Read the model definition and answer for the solid it produces. Units are mm, in the model's axes. Coordinates: 2 decimals unless noted, no trailing zeros. Loops run counter-clockwise (first coordinate to the right, second up) from the corner with the lowest first, then second, coordinate; pieces in that order, holes last. Notation, with made-up numbers: (80, -19) - (123, -19) arc R25 cw to (123, 3) - close; hole circle Ø5 at (52, 84.25). An arc over 180 degrees is marked (long way). Use one line per item in the form item = value.
from build123d import *

# Parameters (mm, degrees)
F0_R     = 83.8
F0_R_2   = 80
F1_DEPTH = 800
F2_W     = 94.3220257759
F2_H     = 124.5050393045
F3_DEPTH = 84.8


with BuildPart() as f1:
    # F0 (on Front) → F1 (new body)
    with BuildSketch(Plane.XZ):
        Circle(F0_R)
        Circle(F0_R_2, mode=Mode.SUBTRACT)
    extrude(amount=F1_DEPTH)

    # F2 (on Top) → F3 (cut, up to face)
    with BuildSketch(Plane.XY):
        with Locations((0, -93.3787897229)):
            Rectangle(F2_W, F2_H)
    extrude(amount=-F3_DEPTH, mode=Mode.SUBTRACT)


solid = f1.part
Item 1: The part is cut by section D-D on y = -451. Give the vertices of the cut face in (x, z).
Results below:
outline = circle Ø167.6 at (0, 0); hole circle Ø160 at (0, 0)
Item 2: For a pull along Y with two mould halves and no side action, classify faces 1 (the flat face through (0, -31.126, -81)), 2 (the flat face through (31, 0, -74)), 3 (the flat face through (0, -155.631, -81)), 4 (the flat face through (31, -800, -74)) as +Y half, -Y half, draft (parallel to the pull), parting line (faces both ways), or undercut.
Results below:
face_1 = undercut
face_2 = +Y half
face_3 = undercut
face_4 = -Y half
Item 3: The part is cut by section C-C on x = 65. Give the vertices of the cut face in (y, z), plus the area to 3 significant figures.
Results below:
outline = (-800, -52.89) - (0, -52.89) - (0, -46.64) - (-800, -46.64) - close; (-800, 46.64) - (0, 46.64) - (0, 52.89) - (-800, 52.89) - close
area = 10,000 mm²
Item 4: The part is cut by section B-B on z = 0. Give the vertices of the cut face in (x, y), plus the area to 3 significant figures.
Results below:
outline = (-83.8, -800) - (-80, -800) - (-80, 0) - (-83.8, 0) - close; (80, -800) - (83.8, -800) - (83.8, 0) - (80, 0) - close
area = 6,080 mm²
Item 5: Find the intervals of material crossed by L1, parallel to Z at x = 0, y = -384; L2, parallel to X at y = -158, z = 3; L3, parallel to Y at x = -39, z = -73, in increasing order.
Results below:
L1 = -83.8 to -80, 80 to 83.8
L2 = -83.75 to -79.94, 79.94 to 83.75
L3 = -800 to -155.63, -31.13 to 0
Item 6: Each of these flat-tipped pins is pushed along its axis until it touches: P1, Ø8, axis at y = -543, z = -39, coming from the +X side; P2, Ø8, axis at y = -105, z = 54, coming from the +X side; P3, Ø4, axis at y = -576.5, z = -66, coming from the -X side. Where does it stop, or does it pass through?
Results below:
P1 = 76.14
P2 = 67.25
P3 = -54.1
Item 7: The part is cut by section A-A on x = 0. Give the vertices of the cut face in (y, z), plus the area to 3 significant figures.
Results below:
outline = (-800, -83.8) - (-155.63, -83.8) - (-155.63, -80) - (-800, -80) - close; (-800, 80) - (0, 80) - (0, 83.8) - (-800, 83.8) - close; (-31.13, -83.8) - (0, -83.8) - (0, -80) - (-31.13, -80) - close
area = 5,610 mm²
